The listing builds one solid part. Answer for the finished solid, in the listing's coordinates (mm). Round coordinates to 2 decimals unless told otherwise and drop trailing zeros. Loops run counter-clockwise (first coordinate to the right, second up) from the corner with the lowest first, then second, coordinate; pieces in that order, holes last. Notation, with made-up numbers: M -29.75,24.25 L 21.25,24.25 A24 ccw 21.25,37.25 Z; hole C -14.75,17 d1. An arc over 180 degrees is marked long. Answer as a JSON object with one key per item and string values.
```python
from build123d import *

# Parameters (mm, degrees)
ESQUISSE1_R             = 15
BOSS_EXTRU_1_DEPTH      = 200
ESQUISSE2_W             = 25
ESQUISSE2_H             = 10
ENL_V_MAT_EXTRU_3_DEPTH = 2


with BuildPart() as part:
    # Esquisse1 → Boss.-Extru.1 (new body)
    with BuildSketch(Plane.XY):
        Circle(ESQUISSE1_R)
    extrude(amount=BOSS_EXTRU_1_DEPTH)

    # Esquisse2 → Enlèv. mat.-Extru.3 (cut)
    with BuildSketch(Plane(origin=(0, 0, 0), x_dir=(-1, 0, 0), z_dir=(0, 0, -1))):
        with Locations((-0.5, 0)):
            Rectangle(ESQUISSE2_W, ESQUISSE2_H)
    extrude(amount=-ENL_V_MAT_EXTRU_3_DEPTH, mode=Mode.SUBTRACT)


solid = part.part
```
Item 1: The part is cut by section A-A (x = -9). Give the vertices of the cut face in (y, z).
Values follow:
{"outline": "M -12,0 L -5,0 L -5,2 L 5,2 L 5,0 L 12,0 L 12,200 L -12,200 Z"}
Item 2: The part is cut by section C-C (y = 3). Give the vertices of the cut face in (x, z), then the cut area to 3 significant figures.
Values follow:
{"outline": "M -14.7,0 L -12,0 L -12,2 L 13,2 L 13,0 L 14.7,0 L 14.7,200 L -14.7,200 Z", "area": "5,830 mm^2"}
Item 3: The part is cut by section B-B (z = 13). Give the vertices of the cut face in (x, y), then the cut area to 3 significant figures.
Values follow:
{"outline": "C 0,0 d30", "area": "707 mm^2"}
Item 4: Flat-ended cylindrical pins translate along their axes: P1, Ø5, axis at y = 4.5, z = 147, coming from the +X side; P2, Ø1, axis at x = -6, z = 81.5, coming from the +Y side; P3, Ø6, axis at y = -10.5, z = 142, coming from the -X side. Find the tip coordinate at first contact, or state that the pin passes through.
Values follow:
{"P1": "x = 14.87", "P2": "y = 13.96", "P3": "x = -12.99"}
Item 5: Straight lines are drawn through the part: line 1 (Z direction, x = 10, y = -1.25); line 2 (X direction, y = -0.5, z = 155.5); line 3 (Y direction, x = -0.75, z = 35). For each, find the intervals that lie inside material, in ascending order.
Values follow:
{"line 1": "2 to 200", "line 2": "-14.99 to 14.99", "line 3": "-14.98 to 14.98"}
Item 6: Determine the mould class of faces 1 (the face through (-14.985, 0.66, 98.6)), 2 (the face through (1, 0, 2)), 3 (the face through (0, -6, 0)) for opening direction X: released by +X, released by -X, zero draft, split by the parting line, or undercut.
Values follow:
{"face 1": "split by the parting line", "face 2": "undercut", "face 3": "zero draft"}
